Input: part model. Units: mm. Frame: model coordinates. A direction names the side the tool comes from. Round coordinates to 2 decimals unless told otherwise and drop trailing zeros. Write each loop counter-clockwise with the first axis right and the second up, starting at its lowest first coordinate (ties: lowest second). Pieces come first, ordered by that corner, then holes. Notation, with made-up numbers: (15, -7.75) - (47, -7.75) arc R30 cw to (47, 14.25) - close; hole circle Ø1 at (-34.75, 38.25). An arc over 180 degrees is marked (long way). Use one line per item in the form item = value.
Autodesk Fusion 360 part; units mm, degrees
sketch "Sketch1" plane through (0, 0, 0) normal (0, 0, 1) x (1, 0, 0)
  line L0 (-15.5, 12.25) -> (15.5, 12.25)
  line L1 (15.5, 12.25) -> (15.5, -12.25)
  line L2 (15.5, -12.25) -> (-15.5, -12.25)
  line L3 (-15.5, -12.25) -> (-15.5, 12.25)
  line L4 (-15.5, 12.25) -> (15.5, -12.25) construction
  line L5 (15.5, 12.25) -> (-15.5, -12.25) construction
  dimension "d1" = 31
  dimension "d2" = 24.5
extrude "Extrude1" add sketch "Sketch1" along normal blind 5.5
shell "Shell1" thickness 1.8 removed faces 1 at (-5.1667, 4.0833, 5.5)
sketch "Sketch2" plane through (0, 0, 5.5) normal (0, 0, 1) x (-1, 0, 0)
  line L0 (13.7, 10.45) -> (13.7, -10.45)
  line L1 (13.7, -10.45) -> (-13.7, -10.45)
  line L2 (-13.7, -10.45) -> (-13.7, 10.45)
  line L3 (-13.7, 10.45) -> (13.7, 10.45)
  line L4 (15.5, 12.25) -> (-15.5, 12.25)
  line L5 (-15.5, 12.25) -> (-15.5, -12.25)
  line L6 (-15.5, -12.25) -> (15.5, -12.25)
  line L7 (15.5, -12.25) -> (15.5, 12.25)
  circle A0 centre (14.4, -11.2) radius 0.84
  line L8 (0, 0) -> (0, -2)
  line L9 (0, 0) -> (4, 0)
  circle A1 centre (-14.4, -11.2) radius 0.84
  circle A2 centre (-14.4, 11.2) radius 0.84
  circle A3 centre (14.4, 11.2) radius 0.84
  dimension "d6" = 1.68
  dimension "d7" = 11.2
  dimension "d8" = 14.4
extrude "Extrude2" add sketch "Sketch2" along normal blind 4 contours A0 | A1 | A2 | A3
fillet "Fillet1" radius 1 1 edges at (15.5, -12.25, 2.75)
fillet "Fillet1" radius 1 1 edges at (15.5, 12.25, 2.75)
fillet "Fillet1" radius 1 1 edges at (-15.5, 12.25, 2.75)
fillet "Fillet1" radius 1 1 edges at (-15.5, -12.25, 2.75)
(1) Cut plane D-D on z = 7. Output: boundary loops of the cut face in (x, y), then the cut area to 3 significant figures.
Derived:
outline = circle Ø1.68 at (-14.4, -11.2); circle Ø1.68 at (-14.4, 11.2); circle Ø1.68 at (14.4, -11.2); circle Ø1.68 at (14.4, 11.2)
area = 8.87 mm^2
(2) First-contact query: pin 1 Ø10 at (x, y) = (7.5, -3) entering from +Z; pin 2 Ø5 at (x, z) = (3, 6) entering from -Y; pin 3 Ø12 at (x, y) = (4.5, 4.5) entering from +Z. Flat tips, straight axial feed; report the tip coordinate or a pass-through.
Derived:
pin_1 = 1.8
pin_2 = -12.25
pin_3 = 5.5
(3) Access query for faces 1 (the face through (-15.199, 11.965, 2.788)), 2 (the face through (15.019, 11.768, 7.472)). Directions: +Z, -Z, +X, -X, +Y, -Y. A direction counts if a zero-diameter tool reaches every point of the face in a straight line with its end or side. Return the directions, or none.
Derived:
face_1 = +Z, -Z, -X, +Y
face_2 = +Z
(4) Cut plane C-C on x = -3.5. Output: boundary loops of the cut face in (y, z).
Derived:
outline = (-12.25, 0) - (12.25, 0) - (12.25, 5.5) - (10.45, 5.5) - (10.45, 1.8) - (-10.45, 1.8) - (-10.45, 5.5) - (-12.25, 5.5) - close
(5) Material intervals for L1, parallel to X at y = 8.75, z = 4; L2, parallel to Y at x = 1, z = 5.25; L3, parallel to Z at x = 13, y = 4.75, sorted ascending.
Derived:
L1 = -15.5 to -13.7, 13.7 to 15.5
L2 = -12.25 to -10.45, 10.45 to 12.25
L3 = 0 to 1.8
(6) Cut plane B-B on y = -3.25. Output: boundary loops of the cut face in (x, z), then the cut area to 3 significant figures.
Derived:
outline = (-15.5, 0) - (15.5, 0) - (15.5, 5.5) - (13.7, 5.5) - (13.7, 1.8) - (-13.7, 1.8) - (-13.7, 5.5) - (-15.5, 5.5) - close
area = 69.1 mm^2
(7) Draft query along Y for faces 3 (the face through (-14, 11, 9.5)), 4 (the face through (0, 0, 1.8)), 5 (the face through (-13.781, -10.632, 7.472)), 6 (the face through (0, -12.25, 3)). Return one class per face: released by +Y, released by -Y, zero draft, split by the parting line, or undercut.
Derived:
face_3 = zero draft
face_4 = undercut
face_5 = undercut
face_6 = released by -Y
(8) Cut plane A-A on z = 2.25. Output: boundary loops of the cut face in (x, y).
Derived:
outline = (-15.5, -11.25) arc R1 ccw to (-14.5, -12.25) - (14.5, -12.25) arc R1 ccw to (15.5, -11.25) - (15.5, 11.25) arc R1 ccw to (14.5, 12.25) - (-14.5, 12.25) arc R1 ccw to (-15.5, 11.25) - close; hole (-13.7, -10.45) - (13.7, -10.45) - (13.7, 10.45) - (-13.7, 10.45) - close
